```python
from build123d import *

# Parameters (mm, degrees)
SKETCH_1_W      = 18
SKETCH_1_H      = 30
EXTRUDE_1_DEPTH = 300
EXTRUDE_2_DEPTH = 20
EXTRUDE_3_DEPTH = 38
SKETCH_6_R      = 0.25
EXTRUDE_4_DEPTH = 0.05
SKETCH_8_R      = 1.5
EXTRUDE_5_DEPTH = 0.1


with BuildPart() as part:
    # 草图1 → 凸台-拉伸1 (new, symmetric)
    with BuildSketch(Plane.XY):
        Rectangle(SKETCH_1_W, SKETCH_1_H)
    extrude(amount=EXTRUDE_1_DEPTH, both=True)

    # 草图3 → 凸台-拉伸2 (add)
    with BuildSketch(Plane.XY.offset(300)):
        Polygon((-9, -15), (-9, -15.05), (9, -15.05), (9, -15), (9, 15), (-9, 15), align=None)
    extrude_2 = extrude(amount=EXTRUDE_2_DEPTH)

    # 镜向1: 凸台-拉伸2 across plane
    add(extrude_2.mirror(Plane.XY))

    # 草图5 → 凸台-拉伸3 (add)
    with BuildSketch(Plane(origin=(19, 0, 0), x_dir=(0, 0, -1), z_dir=(1, 0, 0))):
        Polygon((-165, 25), (-165, -85), (-157, -85), (-150, -58.875644347), (-150, 25), align=None)
    extrude_3 = extrude(amount=-EXTRUDE_3_DEPTH)

    # 镜向2: 凸台-拉伸3 across plane
    add(extrude_3.mirror(Plane.XY))

    # 草图6 → 凸台-拉伸4 (add)
    with BuildSketch(Plane(origin=(0, 15, 0), x_dir=(1, 0, 0), z_dir=(0, 1, 0))):
        with Locations(Location((0, 100, 0), (0, 0, 90))):
            Circle(SKETCH_6_R)
    extrude_4 = extrude(amount=EXTRUDE_4_DEPTH)

    # 镜向3: 凸台-拉伸4 across plane
    add(extrude_4.mirror(Plane.XY))

    # 草图8 → 凸台-拉伸5 (add)
    with BuildSketch(Plane(origin=(0, -26.505017173, 165), x_dir=(1, 0, 0), z_dir=(0, 0, 1))):
        with Locations((0, -53.331799003)):
            Circle(SKETCH_8_R)
    extrude_5 = extrude(amount=EXTRUDE_5_DEPTH)

    # 镜向4: 凸台-拉伸5 across plane
    add(extrude_5.mirror(Plane.XY))


solid = part.part
```
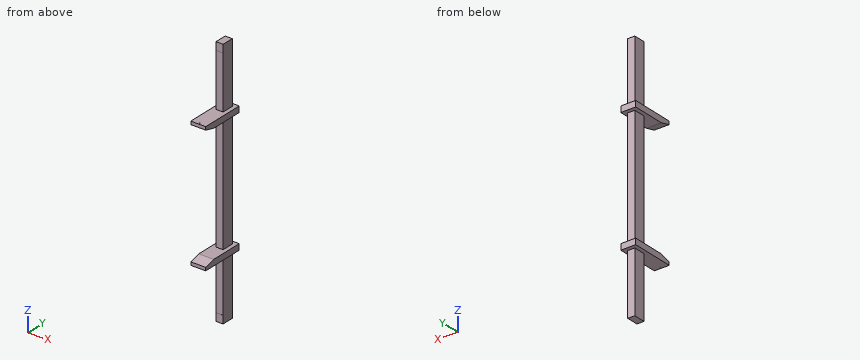
Geometry check sheet. Reference: the model listing, model coordinates, mm. Coordinates: 2 decimals unless noted, no trailing zeros. Order: outer loops, then holes, each group sorted by start corner. A loop starts at its lowest first (then second) coordinate and runs counter-clockwise, first axis right, second up. Notation, with made-up numbers: M 87,-8.75 L 114,-8.75 A23 ccw 114,6.25 Z; hole C 75.25,14.5 d11. An arc over 180 degrees is marked long. Answer as a JSON object with one key per item and string values.
Q1. Scan lines: line 1 (Z direction, x = 11, y = -2); line 2 (Y direction, x = 0.5, z = -111.5); line 3 (X direction, y = 9, z = 17). Record each from-to range of solid material in increasing order.
Results are:
{"line 1": "z = -165 to -150, 150 to 165", "line 2": "y = -15 to 15", "line 3": "x = -9 to 9"}
Q2. Depth check by flat-ended pin: pin 1 Ø12 at (x, z) = (9.5, 252.5) entering from -Y; pin 2 Ø9 at (x, z) = (-0.5, 308) entering from -Y; pin 3 Ø20 at (x, z) = (-2.5, -233.5) entering from +Y. Enter the tip coordinate at first touch or a pass-through.
Results are:
{"pin 1": "stops at y = -15", "pin 2": "stops at y = -15.05", "pin 3": "stops at y = 15"}
Q3. Cross-section at A-A on y = -45.5. Record the cut outline in (x, z), and give its area (3 significant figures).
Results are:
{"outline": "M -19,-165 L 19,-165 L 19,-150 L -19,-150 Z; M -19,150 L 19,150 L 19,165 L -19,165 Z", "area": "1,140 mm²"}
Q4. Cross-section at B-B on z = -15. Record the cut outline in (x, y), and give its area (3 significant figures).
Results are:
{"outline": "M -9,-15 L 9,-15 L 9,15 L -9,15 Z", "area": "540 mm²"}
